```python
from build123d import *

# Parameters (mm, degrees)
SZKIC1_W                    = 100
SZKIC1_H                    = 100
DODANIE_WYCI_GNI_CIE1_DEPTH = 4
SZKIC2_W                    = 97
SZKIC2_H                    = 3
DODANIE_WYCI_GNI_CIE2_DEPTH = 200


with BuildPart() as part:
    # Szkic1 → Dodanie-wyciągnięcie1 (new body)
    with BuildSketch(Plane.XY):
        with Locations((-50, 50)):
            Rectangle(SZKIC1_W, SZKIC1_H)
        with Locations((50, 50)):
            Rectangle(SZKIC1_W, SZKIC1_H)
        with Locations((50, -50)):
            Rectangle(SZKIC1_W, SZKIC1_H)
        with Locations((-50, -50)):
            Rectangle(SZKIC1_W, SZKIC1_H)
    extrude(amount=DODANIE_WYCI_GNI_CIE1_DEPTH)

    # Szkic2 → Dodanie-wyciągnięcie2 (add)
    with BuildSketch(Plane.XY):
        with Locations((-51.5, 1.5)):
            Rectangle(SZKIC2_W, SZKIC2_H)
        with Locations((-51.5, -1.5)):
            Rectangle(SZKIC2_W, SZKIC2_H)
        Polygon((3, 100), (0, 100), (0, 0), (0, -100), (3, -100), align=None)
        Polygon((0, 0), (0, 100), (-3, 100), (-3, 3), (-3, 0), align=None)
        Polygon((0, -100), (0, 0), (-3, 0), (-3, -3), (-3, -100), align=None)
    extrude(amount=DODANIE_WYCI_GNI_CIE2_DEPTH)


solid = part.part
```
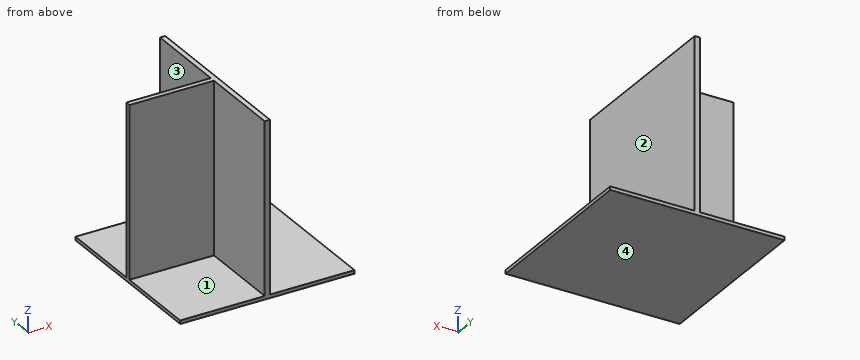
Geometry check sheet. Reference: the model listing, model coordinates, mm. Face numbers are marked on the shaded views. A direction names the side the tool comes from. Give positions to 0.01 mm unless a question says otherwise; leave off trailing zeros. Write each loop counter-clockwise with the first axis right and the second up, starting at its lowest first coordinate (ties: lowest second). Pieces come first, ordered by that corner, then holes. Notation, with made-up numbers: (15.5, 88) - (20.5, 88) arc R7 ccw to (20.5, 99) - close; hole circle Ø7 at (-31, 11.25). An arc over 180 degrees is marked (long way). Use a Markdown table: item, result.
Q1. Go/stop test with flat-tipped pins: P1, Ø1, axis at x = -28.5, z = 123.5, coming from the -Y side; P2, Ø4, axis at y = 40, z = 72.5, coming from the +X side; P3, Ø1.5, axis at y = -50, z = 153, coming from the -X side. Record where each tip stops, or that it passes through.
Computed:
| item | result |
|---|---|
| P1 | stops at y = -3 |
| P2 | stops at x = 3 |
| P3 | stops at x = -3 |
Q2. Section check B-B, the plane y = -72. Enter the section's corners in (x, z).
Computed:
| item | result |
|---|---|
| outline | (-100, 0) - (100, 0) - (100, 4) - (3, 4) - (3, 200) - (-3, 200) - (-3, 4) - (-100, 4) - close |
Q3. Set-up check for the marked faces 1, 2, 3 and 4: record each of +Z, -Z, +X, -X, +Y, -Y from which the full face is reachable in a straight line by a thin tool's end or side.
Computed:
| item | result |
|---|---|
| face 1 | +Z, -X, -Y |
| face 2 | +Z, +X, +Y, -Y |
| face 3 | +Z, -X, +Y |
| face 4 | -Z, +X, -X, +Y, -Y |
Q4. Section check C-C, the plane x = 21.5. Enter the section's corners in (y, z), then the cut area to 3 significant figures.
Computed:
| item | result |
|---|---|
| outline | (-100, 0) - (100, 0) - (100, 4) - (-100, 4) - close |
| area | 800 mm² |
Q5. Section check A-A, the plane z = 56.5. Enter the section's corners in (x, y), then the cut area to 3 significant figures.
Computed:
| item | result |
|---|---|
| outline | (-100, -3) - (-3, -3) - (-3, -100) - (3, -100) - (3, 100) - (-3, 100) - (-3, 3) - (-100, 3) - close |
| area | 1,780 mm² |
Q6. Thickness scan on L1, parallel to Y at x = -17.5, z = 152.5; L2, parallel to Z at x = 64, y = 91.5. Record the ranges inside material, lowest first. Write a range as [from, to].
Computed:
| item | result |
|---|---|
| L1 | y = [-3, 3] |
| L2 | z = [0, 4] |
